Print and shaded views of the part. All mm, measured from the part's lowest x, y and z. A direction names the side the tool comes from. Give positions to 0.01 mm unless a question says otherwise; leave off trailing zeros. Order: outer loops, then holes, each group sorted by start corner. A loop starts at its lowest first (then second) coordinate and runs counter-clockwise, first axis right, second up. Notation, with made-up numbers: (-17, 0) - (4, 0) arc R25 cw to (4, 29) - close; hole circle Ø10 at (-8.75, -34). An arc over 180 degrees is marked (long way). Answer in a Markdown table with one row per item.
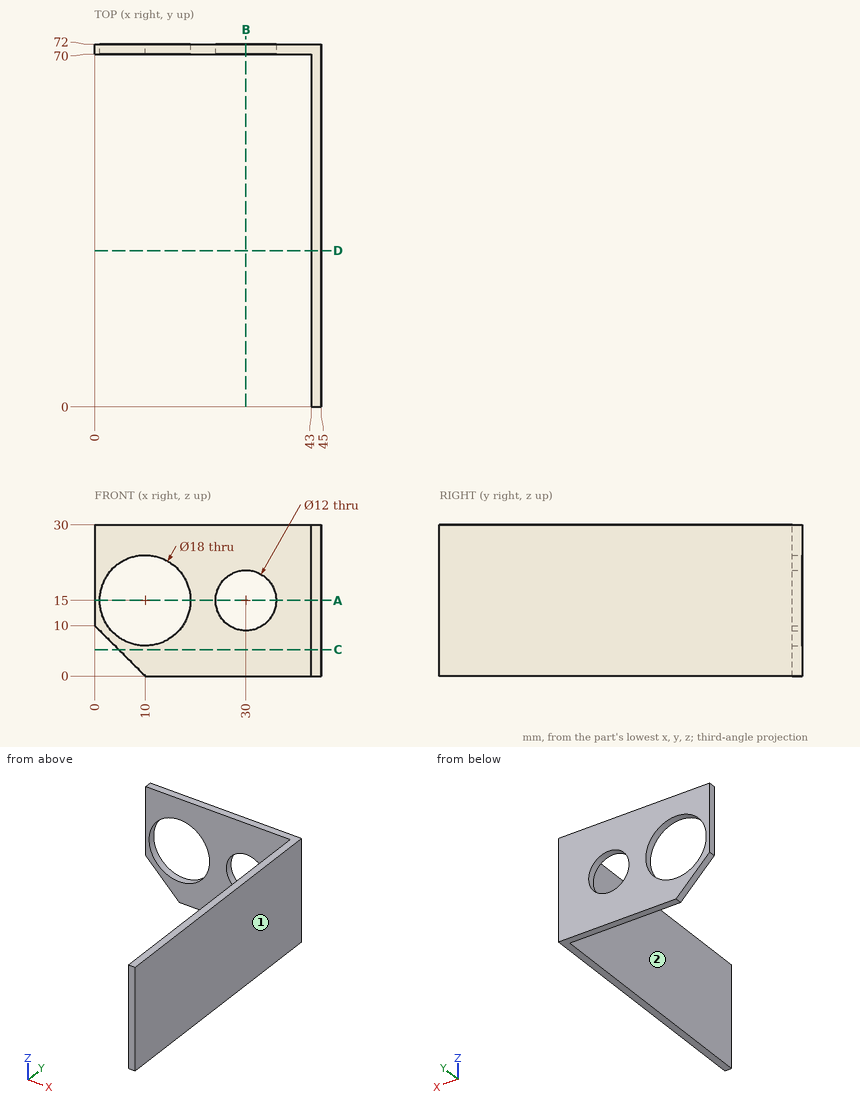
1. Probe line 1 (X direction, y = 70.85, z = 15); line 2 (Z direction, x = 30, y = 71.3); line 3 (X direction, y = 25, z = 3.75). List the from-to ranges inside material, lowest first.
Check result:
| item | result |
|---|---|
| line 1 | x = 0 to 1, 19 to 24, 36 to 45 |
| line 2 | z = 0 to 9, 21 to 30 |
| line 3 | x = 43 to 45 |
2. Drop flat-ended pins along their axis: P1, Ø12, axis at y = 35.5, z = 20.5, coming from the -X side; P2, Ø15, axis at x = 29.5, z = 22, coming from the -Y side. Give the stop position or say it passes through.
Check result:
| item | result |
|---|---|
| P1 | stops at x = 43 |
| P2 | stops at y = 70 |
3. Cut at C-C on z = 5.25. Write the cut outline in (x, y).
Check result:
| item | result |
|---|---|
| outline | (4.75, 70) - (43, 70) - (43, 0) - (45, 0) - (45, 72) - (4.75, 72) - close |
4. Cut at A-A on z = 15. Write the cut outline in (x, y).
Check result:
| item | result |
|---|---|
| outline | (0, 70) - (1, 70) - (1, 72) - (0, 72) - close; (19, 70) - (24, 70) - (24, 72) - (19, 72) - close; (36, 70) - (43, 70) - (43, 0) - (45, 0) - (45, 72) - (36, 72) - close |
5. Cut at D-D on y = 31. Write the cut outline in (x, z).
Check result:
| item | result |
|---|---|
| outline | (43, 0) - (45, 0) - (45, 30) - (43, 30) - close |
6. Which spindle directions (+Z, -Z, +X, -X, +Y, -Y) get a long thin tool onto all of the face, cutting with end or side? Do the marked faces 1 and 2. Say none if no direction does.
Check result:
| item | result |
|---|---|
| face 1 | +Z, -Z, +X, +Y, -Y |
| face 2 | +Z, -Z, -X, -Y |
7. Cut at B-B on x = 30. Write the cut outline in (y, z), and give its area (3 significant figures).
Check result:
| item | result |
|---|---|
| outline | (70, 0) - (72, 0) - (72, 9) - (70, 9) - close; (70, 21) - (72, 21) - (72, 30) - (70, 30) - close |
| area | 36.0 mm² |
